from build123d import *

# Parameters (mm, degrees)
SKIZZE1_W                       = 25
SKIZZE1_H                       = 40
SKIZZE1_R                       = 1.65
AUFSATZ_LINEAR_AUSTRAGEN1_DEPTH = 9
SCHNITT_LINEAR_AUSTRAGEN2_DEPTH = 20
SCHNITT_LINEAR_AUSTRAGEN3_DEPTH = 20
VERRUNDUNG1_R                   = 1


with BuildPart() as part:
    # Skizze1 → Aufsatz-Linear austragen1 (new body)
    with BuildSketch(Plane(origin=(0, 0, 0), x_dir=(1, 0, 0), z_dir=(0, 1, 0))):
        with Locations((12.5, 20)):
            Rectangle(SKIZZE1_W, SKIZZE1_H)
        with Locations(Location((4, 5, 0), (0, 0, 270))):
            Circle(SKIZZE1_R, mode=Mode.SUBTRACT)
        with Locations(Location((21, 5, 0), (0, 0, 270))):
            Circle(SKIZZE1_R, mode=Mode.SUBTRACT)
        with Locations(Location((21, 35, 0), (0, 0, 270))):
            Circle(SKIZZE1_R, mode=Mode.SUBTRACT)
        with Locations(Location((4, 35, 0), (0, 0, 270))):
            Circle(SKIZZE1_R, mode=Mode.SUBTRACT)
    extrude(amount=AUFSATZ_LINEAR_AUSTRAGEN1_DEPTH)

    # Skizze3 → Schnitt-Linear austragen2 (cut)
    with BuildSketch(Plane(origin=(0, 0, -40), x_dir=(-1, 0, 0), z_dir=(0, 0, -1))):
        with BuildLine():
            Line((-15.05, 9), (-9.95, 9))
            ThreePointArc((-9.95, 9), (-12.5, 6.45), (-15.05, 9))
        make_face()
    extrude(amount=-SCHNITT_LINEAR_AUSTRAGEN2_DEPTH, mode=Mode.SUBTRACT)

    # Skizze2 → Schnitt-Linear austragen3 (cut)
    with BuildSketch(Plane.XY):
        with BuildLine():
            Line((17.55, 9), (7.45, 9))
            ThreePointArc((7.45, 9), (12.5, 3.95), (17.55, 9))
        make_face()
    extrude(amount=-SCHNITT_LINEAR_AUSTRAGEN3_DEPTH, mode=Mode.SUBTRACT)

    # Verrundung1
    verrundung1_edges = [part.edges().sort_by_distance(p)[0] for p in [
        (12.5, 6.45, -20),
        (12.5, 3.95, -20),
    ]]
    fillet(verrundung1_edges, radius=VERRUNDUNG1_R)


solid = part.part
CAD build for the part. Positions are in the model's coordinates, mm. A direction names the side the tool comes from. Give positions to 0.01 mm unless a question says otherwise; leave off trailing zeros. Loops run counter-clockwise (first coordinate to the right, second up) from the corner with the lowest first, then second, coordinate; pieces in that order, holes last. Notation, with made-up numbers: M 23.5,69 L 81.5,69 A29 ccw 81.5,99 Z; hole C 10.25,34.25 d11. An arc over 180 degrees is marked long. Answer in a Markdown table with one row per item. Add a question column.
Item 1: Band-saw the part on A-A on x = 21. Give the cut face in (y, z), then the cut area to 3 significant figures.
Item 2: Band-saw the part on C-C on y = 2.75. Give the cut face in (x, z).
Item 3: Drop flat-ended pins along their axis: P1, Ø1.5, axis at y = 7, z = -31.5, coming from the -X side; P2, Ø3, axis at x = 4, z = -5, coming from the -Y side; P3, Ø4.5, axis at x = 12, y = 7.5, coming from the +Z side. Give the stop position or say it passes through.
Item 4: Band-saw the part on B-B on z = -35. Give the cut face in (x, y).
Item 5: Tool access for faces 1 (the face through (12, 0, -20)), 2 (the face through (12.39, 3.95, -9.37)): list every direction of +Z, -Z, +X, -X, +Y, -Y with a clear straight run to the whole face (end or side of a thin tool).
Item 6: Band-saw the part on D-D on z = -23.5. Give the cut face in (x, y).
Item 7: Probe probe 1 along X at (y, z) = (2.75, -35); probe 2 along X at (y, z) = (5.5, -5); probe 3 along Z at (x, y) = (19.75, 3). List the from-to ranges inside material, lowest first.
Item 8: Mould opens along Z. For faces 3 (the face through (12, 4, -40)), 4 (the face through (4.07, 4.44, -36.65)), 5 (the face through (22.636, 4.437, -5.215)), 6 (the face through (12.44, 6.45, -30.63)) say: +Z half, -Z half, draft (parallel to the pull), parting line (faces both ways), or undercut.
Reply:
| question | item | result |
|---|---|---|
| 1 | outline | M 0,-40 L 9,-40 L 9,-36.65 L 0,-36.65 Z; M 0,-33.35 L 9,-33.35 L 9,-6.65 L 0,-6.65 Z; M 0,-3.35 L 9,-3.35 L 9,0 L 0,0 Z |
| 1 | area | 301 mm^2 |
| 2 | outline | M 0,-40 L 25,-40 L 25,0 L 0,0 Z; hole C 4,-35 d3.3; hole C 4,-5 d3.3; hole C 21,-35 d3.3; hole C 21,-5 d3.3 |
| 3 | P1 | stops at x = 0 |
| 3 | P2 | passes through |
| 3 | P3 | stops at z = -20 |
| 4 | outline | M 0,0 L 2.35,0 L 2.35,9 L 0,9 Z; M 5.65,0 L 19.35,0 L 19.35,9 L 15.05,9 A2.55 cw 9.95,9 L 5.65,9 Z; M 22.65,0 L 25,0 L 25,9 L 22.65,9 Z |
| 5 | face 1 | +Z, -Z, +X, -X, -Y |
| 5 | face 2 | +Z, +Y |
| 6 | outline | M 0,0 L 25,0 L 25,9 L 15.05,9 A2.55 cw 9.95,9 L 0,9 Z |
| 7 | probe 1 | x = 0 to 2.35, 5.65 to 19.35, 22.65 to 25 |
| 7 | probe 2 | x = 0 to 2.35, 5.65 to 8.86, 16.14 to 19.35, 22.65 to 25 |
| 7 | probe 3 | z = -40 to -36.08, -33.92 to -6.08, -3.92 to 0 |
| 8 | face 3 | -Z half |
| 8 | face 4 | undercut |
| 8 | face 5 | undercut |
| 8 | face 6 | draft |
